Input: part model. Units: mm. Frame: model coordinates. A direction names the side the tool comes from. Coordinates: 2 decimals unless noted, no trailing zeros. Write each loop counter-clockwise with the first axis right and the second up, starting at its lowest first coordinate (ties: lowest second). Pieces come first, ordered by that corner, then holes. Notation, with made-up numbers: (4, 60.25) - (8, 60.25) arc R21 ccw to (8, 82.25) - close; hole circle Ø6 at (-18, -37.75). An arc over 180 degrees is marked (long way). Put each result on its own line as item: value. Start each with the question number.
1. Line query: line 1 (Y direction, x = 8.5, z = -10.75); line 2 (X direction, y = 8, z = -4.5); line 3 (X direction, y = 20, z = -9.5). Output: solid intervals per line, ascending.
2. Pull-direction query (Y, two-part tool) for faces 1 (the flat face through (36, -0.991, -8)), 2 (the cylindrical face through (-15.87, 17.21, -8.41)), 3 (the cylindrical face through (89.115, 17.258, -8.654)), 4 (the cylindrical face through (87.134, 16.517, -8.415)); classes: released by +Y, released by -Y, zero draft, split by the parting line, or undercut.
3. Access query for faces 5 (the cylindrical face through (35.13, 33.75, -18.06)), 6 (the cylindrical face through (35.13, 33.71, 0.99)), 7 (the flat face through (35, 32.741, -9)), 8 (the cylindrical face through (-17.85, 16.47, -8.65)). Directions: +Z, -Z, +X, -X, +Y, -Y. A direction counts if a zero-diameter tool reaches every point of the face in a straight line with its end or side. Return the directions, or none.
4. Cut plane A-A, the plane x = 35. Return loops of the section in (y, z).
5. Cut plane B-B, the plane z = -7.5. Return loops of the section in (x, y) (3 decimals).
6. Pin query (flat end, axial travel): pin 1 (1 mm diameter, centred on y = 22, z = -2.5, fed in from -X); pin 2 (1 mm diameter, centred on y = 28, z = -4.5, fed in from -X); pin 3 (6 mm diameter, centred on x = 20.5, y = 28, fed in from +Z). Return the tip coordinate at first contact, or that it passes through.
Autodesk Inventor part; units mm, degrees
ref_plane "YZ Plane" through (0, 0, 0) normal (1, 0, 0) x (0, 1, 0)
ref_plane "XZ Plane" through (0, 0, 0) normal (0, 1, 0) x (-1, 0, 0)
ref_plane "XY Plane" through (0, 0, 0) normal (0, 0, 1) x (1, 0, 0)
sketch "Sketch1" plane through (0, 0, 0) normal (0, 0, 1) x (1, 0, 0)
  line L0 (0, 0) -> (71.2633, 0)
  line L1 (71.2633, 33.7312) -> (0, 33.7312)
  arc A0 (0, 33.7312) -> (0, 0) centre (0, 16.8656) ccw
  arc A1 (71.2633, 0) -> (71.2633, 33.7312) centre (71.2633, 16.8656) ccw
  dimension "d2" = 16.8656
  dimension "d3" = 71.2633
sketch "Sketch2" plane through (0, 0, 0) normal (1, 0, 0) x (0, 1, 0)
  arc A0 (0.9906, 0) -> (-0.9906, 0) centre (0, 0) ccw
  line L0 (-0.9906, 0) -> (0.9906, 0) construction
  line L1 (-0.9906, 0) -> (-0.9906, -17.0688)
  line L2 (0.9906, 0) -> (0.9906, -17.0688)
  arc A1 (-0.9906, -17.0688) -> (0.9906, -17.0688) centre (0, -17.0688) ccw
  dimension "d8" = 1.9812
  dimension "d9" = 19.05
sweep "Sweep1" add profiles "Sketch2" path "Sketch1"
properties part number "Short Polycord" material "Rubber, Silicone"
Report:
1. line 1: y = -0.99 to 0.99, 32.74 to 34.72
1. line 2: x = -15.5 to -13.17, 84.43 to 86.76
1. line 3: x = -17.58 to -15.56, 86.83 to 88.84
2. face 1: released by -Y
2. face 2: undercut
2. face 3: split by the parting line
2. face 4: undercut
3. face 5: -Z
3. face 6: +Z
3. face 7: +Z, -Z
3. face 8: +Z, -Z, -X
4. outline: (-0.99, -17.07) arc R0.99 ccw to (0.99, -17.07) - (0.99, 0) arc R0.99 ccw to (-0.99, 0) - close; (32.74, -17.07) arc R0.99 ccw to (34.72, -17.07) - (34.72, 0) arc R0.99 ccw to (32.74, 0) - close
5. outline: (0, -0.991) - (71.263, -0.991) arc R17.856 ccw to (71.263, 34.722) - (0, 34.722) arc R17.856 ccw to start; hole (0, 0.991) - (71.263, 0.991) arc R15.875 ccw to (71.263, 32.741) - (0, 32.741) arc R15.875 ccw to start
6. pin 1: stops at x = -17.24
6. pin 2: stops at x = -14.34
6. pin 3: passes through
